Geometry: final body of the model. Coordinates: model frame, mm. A direction names the side the tool comes from. Coordinates: 2 decimals unless noted, no trailing zeros. Write each loop counter-clockwise with the first axis right and the second up, starting at its lowest first coordinate (ties: lowest second). Pieces come first, ordered by that corner, then holes.
from build123d import *

# Parameters (mm, degrees)
BOSS_EXTRUDE1_DEPTH = 135
CUT_EXTRUDE1_REACH  = 151.833


with BuildPart() as part:
    # Sketch2 → Boss-Extrude1 (new body)
    with BuildSketch(Plane(origin=(0, 0, 0), x_dir=(0, 0, 1), z_dir=(1, 0, 0))):
        Polygon((-9, 23), (9, 23), (9, 0), (30, 0), (30, -52), (21, -52), (0, -15.626933041), (-21, -52), (-30, -52), (-30, 0), (-9, 0), align=None)
    extrude(amount=BOSS_EXTRUDE1_DEPTH)

    # Sketch3 → Cut-Extrude1 (cut, up to next)
    with BuildSketch(Plane(origin=(0, 0, -9), x_dir=(-1, 0, 0), z_dir=(0, 0, -1)), mode=Mode.PRIVATE) as cut_extrude1_sk1:
        Polygon((-65, -9), (-79, -23), (-51, -23), align=None)
    cut_extrude1_tool1 = extrude(cut_extrude1_sk1.sketch, amount=-CUT_EXTRUDE1_REACH, mode=Mode.PRIVATE) & part.part
    # Sketch3 → Cut-Extrude1 (cut, up to next)
    with BuildSketch(Plane(origin=(0, 0, -9), x_dir=(-1, 0, 0), z_dir=(0, 0, -1)), mode=Mode.PRIVATE) as cut_extrude1_sk2:
        Polygon((-93, -9), (-107, -23), (-79, -23), align=None)
    cut_extrude1_tool2 = extrude(cut_extrude1_sk2.sketch, amount=-CUT_EXTRUDE1_REACH, mode=Mode.PRIVATE) & part.part
    # Sketch3 → Cut-Extrude1 (cut, up to next)
    with BuildSketch(Plane(origin=(0, 0, -9), x_dir=(-1, 0, 0), z_dir=(0, 0, -1)), mode=Mode.PRIVATE) as cut_extrude1_sk3:
        Polygon((-121, -9), (-135, -23), (-107, -23), align=None)
    cut_extrude1_tool3 = extrude(cut_extrude1_sk3.sketch, amount=-CUT_EXTRUDE1_REACH, mode=Mode.PRIVATE) & part.part
    # Sketch3 → Cut-Extrude1 (cut, up to next)
    with BuildSketch(Plane(origin=(0, 0, -9), x_dir=(-1, 0, 0), z_dir=(0, 0, -1)), mode=Mode.PRIVATE) as cut_extrude1_sk4:
        Polygon((-37, -9), (-51, -23), (-23, -23), align=None)
    cut_extrude1_tool4 = extrude(cut_extrude1_sk4.sketch, amount=-CUT_EXTRUDE1_REACH, mode=Mode.PRIVATE) & part.part
    add(cut_extrude1_tool1.solids().sort_by_distance((65, -18.333333, -9))[0], mode=Mode.SUBTRACT)
    add(cut_extrude1_tool2.solids().sort_by_distance((93, -18.333333, -9))[0], mode=Mode.SUBTRACT)
    add(cut_extrude1_tool3.solids().sort_by_distance((121, -18.333333, -9))[0], mode=Mode.SUBTRACT)
    add(cut_extrude1_tool4.solids().sort_by_distance((37, -18.333333, -9))[0], mode=Mode.SUBTRACT)


solid = part.part
Item 1: Section A-A, the plane y = -13. Output: boundary loops of the cut face in (x, z), plus the area to 3 significant figures.
Derived:
outline: (0, -9) - (33, -9) - (33, 9) - (0, 9) - close; (41, -9) - (61, -9) - (61, 9) - (41, 9) - close; (69, -9) - (89, -9) - (89, 9) - (69, 9) - close; (97, -9) - (117, -9) - (117, 9) - (97, 9) - close; (125, -9) - (135, -9) - (135, 9) - (125, 9) - close
area: 1,850 mm2
Item 2: Section B-B, the plane x = 15. Output: boundary loops of the cut face in (y, z).
Derived:
outline: (-23, -9) - (0, -9) - (0, -30) - (52, -30) - (52, -21) - (15.63, 0) - (52, 21) - (52, 30) - (0, 30) - (0, 9) - (-23, 9) - close
Item 3: Material intervals for probe 1 along X at (y, z) = (-17.5, -0.5); probe 2 along Z at (x, y) = (122.5, -7.5); probe 3 along Z at (x, y) = (98, 21), sorted ascending.
Derived:
probe 1: x = 0 to 28.5, 45.5 to 56.5, 73.5 to 84.5, 101.5 to 112.5, 129.5 to 135
probe 2: z = -9 to 9
probe 3: z = -30 to -3.1, 3.1 to 30
Item 4: Pull-direction query (Z, two-part tool) for faces 1 (the flat face through (67, 26, 30)), 2 (the flat face through (44, -16, 0)), 3 (the flat face through (66.555, 33.559, -10.353)); classes: released by +Z, released by -Z, zero draft, split by the parting line, or undercut.
Derived:
face 1: released by +Z
face 2: zero draft
face 3: undercut
Item 5: Section D-D, the plane z = -4. Output: boundary loops of the cut face in (x, y), plus the area to 3 significant figures.
Derived:
outline: (0, -23) - (23, -23) - (37, -9) - (51, -23) - (65, -9) - (79, -23) - (93, -9) - (107, -23) - (121, -9) - (135, -23) - (135, 22.56) - (0, 22.56) - close
area: 5,370 mm2
Item 6: Section C-C, the plane y = 32.5. Output: boundary loops of the cut face in (x, z), plus the area to 3 significant figures.
Derived:
outline: (0, -30) - (135, -30) - (135, -9.74) - (0, -9.74) - close; (0, 9.74) - (135, 9.74) - (135, 30) - (0, 30) - close
area: 5,470 mm2
Item 7: Set-up query: faces 4 (the flat face through (128, -16, 0)), 5 (the flat face through (67, -9, -9)), 6 (the flat face through (66.55, 34.07, 10.65)). Return all of +Z, -Z, +X, -X, +Y, -Y with unobstructed straight access to the full face (end or side cutting, diameter ignored); none if empty.
Derived:
face 4: +Z, -Z, -Y
face 5: -Z, +X, -X, -Y
face 6: +X, -X, +Y
Item 8: Pin query (flat end, axial travel): pin 1 (12 mm diameter, centred on x = 92, z = 2, fed in from -Y); pin 2 (7 mm diameter, centred on x = 99, y = -14.5, fed in from -Z); pin 3 (6.5 mm diameter, centred on x = 79, z = -16, fed in from -Y). Return the tip coordinate at first contact, or that it passes through.
Derived:
pin 1: stops at y = -16
pin 2: stops at z = -9
pin 3: stops at y = 0
